Source: CAD feature listing. Evaluate the final solid. Frame: model axes, mm. Give positions to 0.01 mm unless a question says otherwise; leave off trailing zeros. Write each loop counter-clockwise with the first axis right and the second up, starting at its lowest first coordinate (ties: lowest second). Pieces come first, ordered by that corner, then holes. Notation, with made-up numbers: (7.25, 87.5) -> (22.25, 87.5) arc R23 ccw to (22.25, 95.5) -> close; hole circle Ø9 at (-5, 25.5). An arc over 180 degrees is marked (long way). Use one line per item in the form item = value. Start each with the question number.
(1) Cut plane A-A, the plane x = -12. Output: boundary loops of the cut face in (y, z).
(2) Cut plane C-C, the plane y = 1.25. Output: boundary loops of the cut face in (x, z), and give its area (3 significant figures).
(3) Material intervals for line 1 along X through (y, z) = (0.8, -4); line 2 along Z through (x, y) = (-4, 1.05); line 3 along X through (y, z) = (0.35, -3), sorted ascending. Write a range as from..to.
(4) Cut plane D-D, the plane x = -5.25. Output: boundary loops of the cut face in (y, z), and give its area (3 significant figures).
(5) Draft query along X for faces 1 (the face through (-8, 0, -4)), 2 (the face through (-2.57, 0.76, -4.45)), 3 (the face through (-15.75, 1, -4)). Return one class per face: pulls with the +X half, pulls with the -X half, needs draft (parallel to the pull), parting line crosses it, or undercut.
(6) Cut plane B-B, the plane z = -3.5. Output: boundary loops of the cut face in (x, y), and give its area (3 significant figures).
(7) First-contact query: P1, Ø2.5, axis at x = -12, z = -4, coming from the -Y side; P2, Ø3, axis at x = -3, z = -3.5, coming from the -Y side. Flat tips, straight axial feed; report the tip coordinate or a pass-through.
Autodesk Inventor part; units mm, degrees
ref_plane "YZ Plane" through (0, 0, 0) normal (1, 0, 0) x (0, 1, 0)
ref_plane "XZ Plane" through (0, 0, 0) normal (0, 1, 0) x (-1, 0, 0)
ref_plane "XY Plane" through (0, 0, 0) normal (0, 0, 1) x (1, 0, 0)
sketch "Sketch1" plane through (0, 0, 0) normal (0, 1, 0) x (-1, 0, 0)
  line L0 (0, 0) -> (16, 0)
  line L1 (16, 0) -> (16, -8)
  line L2 (16, -8) -> (0, -8)
  line L3 (0, -8) -> (0, 0)
  dimension "d0" = 16
  dimension "d1" = 8
extrude "Extrusion1" add sketch "Sketch1" along normal blind 1.5
sketch "Sketch2" plane through (0, 1.5, 0) normal (0, 1, 0) x (1, 0, 0)
  circle A0 centre (-4, 4) radius 1.5
  circle A1 centre (-12, 4) radius 1.5
  point P0 (0, 0)
  point P1 (-16, 0)
  dimension "d4" = 3
  dimension "d5" = 3
extrude "Extrusion2" cut sketch "Sketch2" against normal blind 1.5
sketch "Sketch3" plane through (0, 1.5, 0) normal (0, 1, 0) x (1, 0, 0)
  line L0 (-16, 0) -> (0, 0)
  line L1 (0, 0) -> (0, 8)
  line L2 (-16, 0) -> (0, 0)
  line L3 (0, 0) -> (0, 8)
  line L4 (0, 8) -> (-16, 8)
  line L5 (-16, 8) -> (-16, 0)
  line L6 (0, 0) -> (-0.25, 0)
  line L7 (-0.25, 0) -> (-0.25, 8)
  line L8 (0, 0) -> (0, 0.25)
  line L9 (0, 0.25) -> (-16, 0.25)
  line L10 (-16, 0) -> (-15.75, 0)
  line L11 (-15.75, 0) -> (-15.75, 8)
  line L12 (-16, 8) -> (-16, 7.75)
  line L13 (-16, 7.75) -> (-0.25, 7.75)
  point P0 (-0.25, 0.25)
  point P1 (-15.75, 0.25)
  point P2 (-15.75, 7.75)
  dimension "d8" = 0.25
  dimension "d9" = 0.25
  dimension "d10" = 0.25
  dimension "d11" = 0.25
extrude "Extrusion3" cut sketch "Sketch3" against normal blind 1.5 contours L5 L9 L11 L0 | L11 L9 L7 L0 | L5 L13 L11 L9 | L7 L9 L1 L0 | L5 L4 L11 L13 | L7 L4 L1 L9 | L11 L4 L7 L13
properties part number "connector"
Geometry says:
q1.outline = (0, -7.75) -> (1.5, -7.75) -> (1.5, -5.5) -> (0, -5.5) -> close; (0, -2.5) -> (1.5, -2.5) -> (1.5, -0.25) -> (0, -0.25) -> close
q2.outline = (-15.75, -7.75) -> (-0.25, -7.75) -> (-0.25, -0.25) -> (-15.75, -0.25) -> close; hole circle Ø3 at (-12, -4); hole circle Ø3 at (-4, -4)
q2.area = 102 mm^2
q3.line_1 = -15.75..-13.5, -10.5..-5.5, -2.5..-0.25
q3.line_2 = -7.75..-5.5, -2.5..-0.25
q3.line_3 = -15.75..-13.12, -10.88..-5.12, -2.88..-0.25
q4.outline = (0, -7.75) -> (1.5, -7.75) -> (1.5, -4.83) -> (0, -4.83) -> close; (0, -3.17) -> (1.5, -3.17) -> (1.5, -0.25) -> (0, -0.25) -> close
q4.area = 8.76 mm^2
q5.face_1 = needs draft
q5.face_2 = undercut
q5.face_3 = pulls with the -X half
q6.outline = (-15.75, 0) -> (-13.41, 0) -> (-13.41, 1.5) -> (-15.75, 1.5) -> close; (-10.59, 0) -> (-5.41, 0) -> (-5.41, 1.5) -> (-10.59, 1.5) -> close; (-2.59, 0) -> (-0.25, 0) -> (-0.25, 1.5) -> (-2.59, 1.5) -> close
q6.area = 14.8 mm^2
q7.P1 = through
q7.P2 = 0
